Here's the drawing with two shaded views (mm, measured from the low corner). I have some questions. Coordinates: 2 decimals unless noted, no trailing zeros. Write each loop counter-clockwise with the first axis right and the second up, starting at its lowest first coordinate (ties: lowest second). Pieces come first, ordered by that corner, then holes.
Item 1: I want a section at C-C on y = 1.7. Please give me the cut outline in (x, z), then the cut area to 3 significant figures.
Item 2: I want a section at A-A on x = 73.5. Please give me the cut outline in (y, z) (1 decimal), then the cut area to 3 significant figures.
Item 3: I want a section at B-B on x = 98.9. Please give me the cut outline in (y, z) (1 decimal).
Item 4: For P1, Ø4.5, axis at x = 73.5, z = 29.54, coming from the -Y side; P2, Ø1.5, axis at x = 35.5, y = 1.5, coming from the -Z side, each with a flat end and sliding along its axis, tell me the tip position at first contact or that it passes through.
Item 5: If I drill on probe 1 along Z at (x, y) = (98.9, 1.8); probe 2 along X at (y, z) = (3, 51); probe 3 along X at (y, z) = (2.4, 28) (1 decimal), over which ranges is the centre line in solid material (lowest first)?
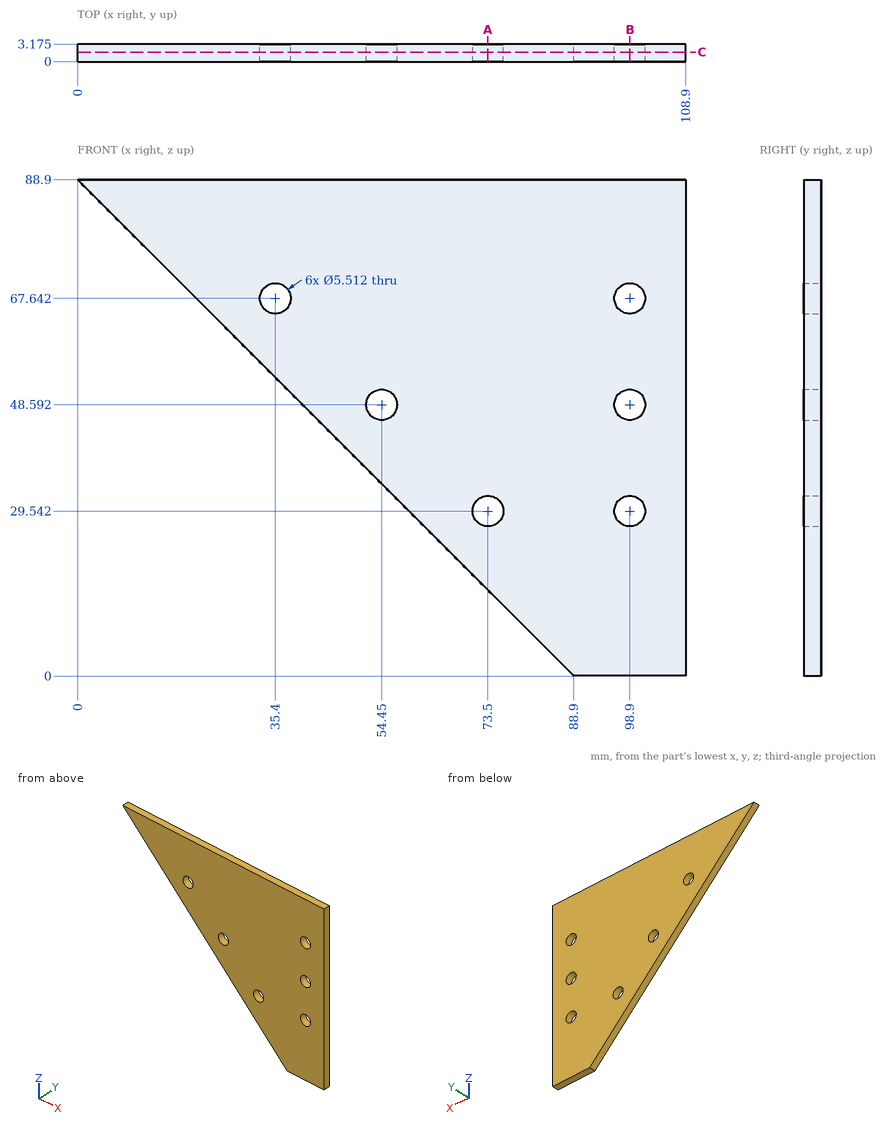
Response values:
1. outline: (0, 88.9) - (88.9, 0) - (108.9, 0) - (108.9, 88.9) - close; hole circle Ø5.51 at (35.4, 67.64); hole circle Ø5.51 at (54.45, 48.59); hole circle Ø5.51 at (73.5, 29.54); hole circle Ø5.51 at (98.9, 29.54); hole circle Ø5.51 at (98.9, 48.59); hole circle Ø5.51 at (98.9, 67.64)
1. area: 5,590 mm2
2. outline: (0, 15.4) - (3.2, 15.4) - (3.2, 26.8) - (0, 26.8) - close; (0, 32.3) - (3.2, 32.3) - (3.2, 88.9) - (0, 88.9) - close
2. area: 216 mm2
3. outline: (0, 0) - (3.2, 0) - (3.2, 26.8) - (0, 26.8) - close; (0, 32.3) - (3.2, 32.3) - (3.2, 45.8) - (0, 45.8) - close; (0, 51.3) - (3.2, 51.3) - (3.2, 64.9) - (0, 64.9) - close; (0, 70.4) - (3.2, 70.4) - (3.2, 88.9) - (0, 88.9) - close
4. P1: passes through
4. P2: stops at z = 52.65
5. probe 1: z = 0 to 26.79, 32.3 to 45.84, 51.35 to 64.89, 70.4 to 88.9
5. probe 2: x = 37.9 to 53.11, 55.79 to 97.56, 100.24 to 108.9
5. probe 3: x = 60.9 to 71.2, 75.8 to 96.6, 101.2 to 108.9
